Can you work these out from the model? Positions are in its coordinate system, mm. Face numbers are marked on the shaded views. Give positions to 0.01 mm unless a question says otherwise; leave off trailing zeros. Loops run counter-clockwise (first coordinate to the right, second up) from the corner with the lowest first, then second, coordinate; pieces in that order, holes last. Notation, with made-up numbers: M 48.5,77 L 52.5,77 A22 cw 52.5,94 Z; hole C 43,-36.5 d2. An arc over 180 degrees is marked long. Put each result on its own line as item: value. Start each with the question number.
1) If we mould it in two halves opening along X, with no side actions, what happens to the marked faces 1, 2 and 3? For each: +X half, -X half, draft (parallel to the pull), parting line (faces both ways), or undercut.
2) For P1, Ø1.5, axis at x = -3, z = 2, coming from the +Y side; P2, Ø4, axis at x = 3, z = 2.5, coming from the -Y side; P3, Ø4, axis at x = -0.5, y = -1.5, coming from the +Z side, each with a flat end and sliding along its axis, tell me the tip position at first contact or that it passes through.
3) Imagine slicing it at A-A (x = 0). Write out the boundary of the cut face in (y, z), then the cut area to 3 significant figures.
4) Imagine slicing it at C-C (z = 4). Write out the boundary of the cut face in (x, y).
5) Please list where these lines run through material, in increasing order: line 1 along Y through (x, z) = (0, 6.25); line 2 along Z through (x, y) = (-0.75, -0.5); line 3 along X through (y, z) = (-1, 1). Write a range as from..to.
Autodesk Inventor part; units mm, degrees
ref_plane "YZ Plane" through (0, 0, 0) normal (1, 0, 0) x (0, 1, 0)
ref_plane "XZ Plane" through (0, 0, 0) normal (0, 1, 0) x (-1, 0, 0)
ref_plane "XY Plane" through (0, 0, 0) normal (0, 0, 1) x (1, 0, 0)
sketch "Szkic1" plane through (0, 0, 0) normal (0, 0, 1) x (1, 0, 0)
  circle A0 centre (0, 0) radius 4.5
  dimension "d0" = 9
extrude "Wyciągnięcie proste1" add sketch "Szkic1" along normal blind 8
shell "Skorupa1" thickness 0.5 removed faces 1 at (0.1808, 1.316, 8)
thread "Gwint1"
fillet "Zaokrąglenie1" radius 1 1 edges at (-4.5, 0, 0)
properties part number "Nakrętka_wentyla" material "Aluminium AW-7020"
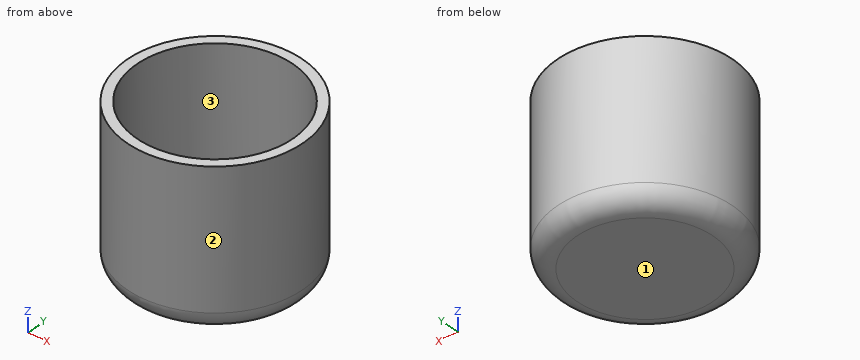
Recorded:
1. face 1: draft
1. face 2: parting line
1. face 3: undercut
2. P1: y = 3.9
2. P2: y = -4.39
2. P3: z = 0.5
3. outline: M -4.5,1 A1 ccw -3.5,0 L 3.5,0 A1 ccw 4.5,1 L 4.5,8 L 4,8 L 4,0.5 L -4,0.5 L -4,8 L -4.5,8 Z
3. area: 11.6 mm²
4. outline: C 0,0 d9; hole C 0,0 d8
5. line 1: -4.5..-4, 4..4.5
5. line 2: 0..0.5
5. line 3: -4.39..-3.87, 3.87..4.39
